Check sheet for the modelled part. Datum: model origin and axes. Units: mm. Face numbers are marked on the shaded views. A direction names the side the tool comes from. Round coordinates to 2 decimals unless told otherwise and drop trailing zeros. Order: outer loops, then holes, each group sorted by start corner. A loop starts at its lowest first (then second) coordinate and runs counter-clockwise, first axis right, second up. Notation, with made-up numbers: (83.5, 3.5) -> (128.5, 3.5) arc R17 cw to (128.5, 20.5) -> close; hole circle Ø9 at (36.5, 71). An arc over 180 degrees is marked (long way). Answer in a Markdown table with one row per item. Add a question column.
1. Access from +Z, -Z, +X, -X, +Y, -Y to the whole of each face (thin tool, end or side, straight path). Record for the marked faces 1, 2 and 3.
2. Material ranges on L1, parallel to Z at x = -81, y = 10; L2, parallel to Y at x = 49, z = -90; L3, parallel to Z at x = 1.5, y = 24.5, recorded low to high. Write a range as from..to.
3. Depth check by flat-ended pin: P1, Ø3, axis at y = 27, z = -88.5, coming from the +X side; P2, Ø4, axis at y = 7, z = -69, coming from the +X side; P3, Ø12, axis at y = 12, z = 5, coming from the -X side; P4, Ø12, axis at x = -26.5, z = -37, coming from the -Y side. Enter the tip coordinate at first touch or a pass-through.
4. Sectioned sample at B-B, the plane z = -35. Record the boundary of the cut face in (x, y).
5. Draft check along Z on the marked faces 4, 5 and 6. Enter one of: +Z half, -Z half, draft (parallel to the pull), parting line (faces both ways), or undercut.
6. Sectioned sample at C-C, the plane x = -36.5. Record the boundary of the cut face in (y, z), then the cut area to 3 significant figures.
7. Sectioned sample at A-A, the plane x = 41.5. Count the separate pieces of the cut face and the enclosed holes in it, then the cut area to 3 significant figures.
```python
from build123d import *

# Parameters (mm, degrees)
ESQUISSE2_W             = 200
ESQUISSE2_H             = 200
BASE_DEPTH              = 40
ESQUISSE3_R             = 15
BLOC_MOTEUR_1_DEPTH     = 80
ESQUISSE4_W             = 10
ESQUISSE4_H             = 22.360679774
ACCES_MOTEUR_DEPTH      = 37
ESQUISSE6_R             = 16.01
BLOC_MOTEUR_2_DEPTH     = 37
ESQUISSE7_R             = 2.5
VIS_MOTEUR_DEPTH        = 147.969384567
ESQUISSE8_R             = 45
VIDE_ROUE_DEPTH         = 5
ESQUISSE9_W             = 10
ESQUISSE9_H             = 40
VIDE_GUIDAGE_TIGE_DEPTH = 10
ESQUISSE10_R            = 2.5
TROU_VIS_DEPTH          = 100
ESQUISSE11_R            = 2.5
VIDE_PATIN_DEPTH        = 147.969384567


with BuildPart() as part:
    # Esquisse2 → BASE (new body)
    with BuildSketch(Plane(origin=(0, 0, 0), x_dir=(1, 0, 0), z_dir=(0, 1, 0))):
        Rectangle(ESQUISSE2_W, ESQUISSE2_H)
    extrude(amount=BASE_DEPTH)

    # Esquisse3 → BLOC MOTEUR 1. (cut)
    with BuildSketch(Plane(origin=(100, 0, 0), x_dir=(0, 0, -1), z_dir=(1, 0, 0))):
        with Locations((35, 10)):
            Circle(ESQUISSE3_R)
    bloc_moteur_1 = extrude(amount=-BLOC_MOTEUR_1_DEPTH, mode=Mode.SUBTRACT)

    # Esquisse4 → ACCES MOTEUR (cut)
    with BuildSketch(Plane.XZ):
        with Locations((25, -35)):
            Rectangle(ESQUISSE4_W, ESQUISSE4_H)
    acces_moteur = extrude(amount=-ACCES_MOTEUR_DEPTH, mode=Mode.SUBTRACT)

    # Esquisse6 → BLOC MOTEUR 2 (cut)
    with BuildSketch(Plane(origin=(100, 0, 0), x_dir=(0, 0, -1), z_dir=(1, 0, 0))):
        with Locations((35, 10)):
            Circle(ESQUISSE6_R)
    bloc_moteur_2 = extrude(amount=-BLOC_MOTEUR_2_DEPTH, mode=Mode.SUBTRACT)

    # SYM BLOC MOTEUR: BLOC MOTEUR 1., ACCES MOTEUR, BLOC MOTEUR 2 across plane
    add(bloc_moteur_1.mirror(Plane(origin=(0, 0, 0), x_dir=(0, 0, 1), z_dir=(1, 0, 0))), mode=Mode.SUBTRACT)
    add(acces_moteur.mirror(Plane(origin=(0, 0, 0), x_dir=(0, 0, 1), z_dir=(1, 0, 0))), mode=Mode.SUBTRACT)
    add(bloc_moteur_2.mirror(Plane(origin=(0, 0, 0), x_dir=(0, 0, 1), z_dir=(1, 0, 0))), mode=Mode.SUBTRACT)

    # Esquisse7 → VIS MOTEUR (cut, through all)
    with BuildSketch(Plane.XZ):
        with Locations(Location((-81.5, -12.497196314, 0), (0, 0, 270))):
            Circle(ESQUISSE7_R)
        with Locations(Location((-41.5, -13.819660113, 0), (0, 0, 270))):
            Circle(ESQUISSE7_R)
        with Locations(Location((-41.5, -56.180339887, 0), (0, 0, 270))):
            Circle(ESQUISSE7_R)
        with Locations(Location((-81.5, -57.502803686, 0), (0, 0, 270))):
            Circle(ESQUISSE7_R)
    vis_moteur = extrude(amount=-VIS_MOTEUR_DEPTH, mode=Mode.SUBTRACT)

    # SYM VIS: VIS MOTEUR across plane
    add(vis_moteur.mirror(Plane(origin=(0, 0, 0), x_dir=(0, 0, 1), z_dir=(1, 0, 0))), mode=Mode.SUBTRACT)

    # Esquisse8 → VIDE ROUE (cut)
    with BuildSketch(Plane(origin=(100, 0, 0), x_dir=(0, 0, -1), z_dir=(1, 0, 0))):
        with Locations((34.831239624, 10.203988641)):
            Circle(ESQUISSE8_R)
    vide_roue = extrude(amount=-VIDE_ROUE_DEPTH, mode=Mode.SUBTRACT)

    # Esquisse9 → VIDE GUIDAGE TIGE (cut)
    with BuildSketch(Plane(origin=(100, 0, 0), x_dir=(0, 0, -1), z_dir=(1, 0, 0))):
        with Locations((90, 20)):
            Rectangle(ESQUISSE9_W, ESQUISSE9_H)
        with Locations((-90, 20)):
            Rectangle(ESQUISSE9_W, ESQUISSE9_H)
    vide_guidage_tige = extrude(amount=-VIDE_GUIDAGE_TIGE_DEPTH, mode=Mode.SUBTRACT)

    # Esquisse10 → TROU VIS (cut)
    with BuildSketch(Plane(origin=(90, 0, 0), x_dir=(0, 0, -1), z_dir=(1, 0, 0))):
        with Locations((-90, 35)):
            Circle(ESQUISSE10_R)
        with Locations((-90, 25)):
            Circle(ESQUISSE10_R)
        with Locations(Location((90, 25, 0), (0, 0, 180))):
            Circle(ESQUISSE10_R)
        with Locations(Location((90, 35, 0), (0, 0, 180))):
            Circle(ESQUISSE10_R)
        with Locations((-90, 15)):
            Circle(ESQUISSE10_R)
        with Locations(Location((90, 15, 0), (0, 0, 180))):
            Circle(ESQUISSE10_R)
    trou_vis = extrude(amount=-TROU_VIS_DEPTH, mode=Mode.SUBTRACT)

    # SYM - ROUE - TIGE: VIDE ROUE, VIDE GUIDAGE TIGE, TROU VIS across plane
    add(vide_roue.mirror(Plane(origin=(0, 0, 0), x_dir=(0, 0, 1), z_dir=(1, 0, 0))), mode=Mode.SUBTRACT)
    add(vide_guidage_tige.mirror(Plane(origin=(0, 0, 0), x_dir=(0, 0, 1), z_dir=(1, 0, 0))), mode=Mode.SUBTRACT)
    add(trou_vis.mirror(Plane(origin=(0, 0, 0), x_dir=(0, 0, 1), z_dir=(1, 0, 0))), mode=Mode.SUBTRACT)

    # Esquisse11 → VIDE PATIN (cut, through all)
    with BuildSketch(Plane.XZ):
        with Locations(Location((-50, 70, 0), (0, 0, 270))):
            Circle(ESQUISSE11_R)
        with Locations(Location((50, 70, 0), (0, 0, 90))):
            Circle(ESQUISSE11_R)
    extrude(amount=-VIDE_PATIN_DEPTH, mode=Mode.SUBTRACT)


solid = part.part
```
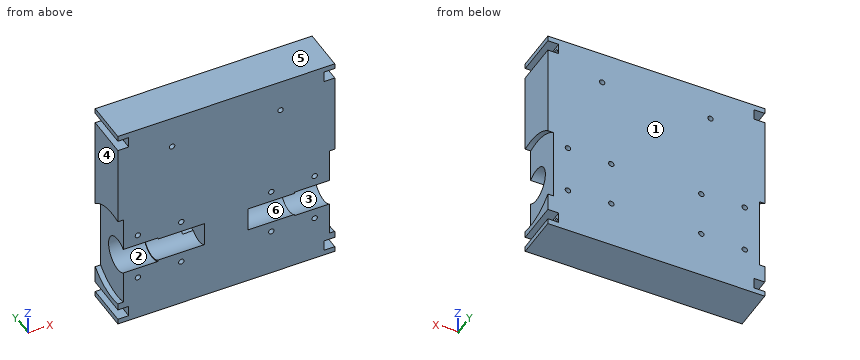
Answer key:
| question | item | result |
|---|---|---|
| 1 | face 1 | +Z, -Z, +X, -X, +Y |
| 1 | face 2 | -X |
| 1 | face 3 | +X |
| 2 | L1 | z = -100..-59.95, -55.05..-51.01, -18.99..-14.95, -10.05..100 |
| 2 | L2 | y = 0..12.5, 17.5..22.5, 27.5..32.5, 37.5..40 |
| 2 | L3 | z = -100..-92.45, -87.55..87.55, 92.45..100 |
| 3 | P1 | stops at x = 90 |
| 3 | P2 | stops at x = 95 |
| 3 | P3 | stops at x = -100 |
| 3 | P4 | stops at y = 23.33 |
| 4 | outline | (-95, 26.01) -> (-63, 26.01) -> (-63, 25) -> (-30, 25) -> (-30, 37) -> (-20, 37) -> (-20, 0) -> (20, 0) -> (20, 37) -> (30, 37) -> (30, 25) -> (63, 25) -> (63, 26.01) -> (95, 26.01) -> (95, 40) -> (-95, 40) -> close |
| 5 | face 4 | draft |
| 5 | face 5 | +Z half |
| 5 | face 6 | undercut |
| 6 | outline | (0, -100) -> (40, -100) -> (40, 100) -> (0, 100) -> (0, -23.82) arc R15 cw (long way) to (0, -46.18) -> close; hole circle Ø5 at (15, -90); hole circle Ø5 at (15, 90); hole circle Ø5 at (25, -90); hole circle Ø5 at (25, 90); hole circle Ø5 at (35, -90); hole circle Ø5 at (35, 90) |
| 6 | area | 7,250 mm² |
| 7 | separate pieces | 3 |
| 7 | enclosed holes | 6 |
| 7 | area | 6,850 mm² |
